Geometry: see drawing. Coordinates: mm, zero at the bounding-box minimum. Coordinates: 2 decimals unless noted, no trailing zeros. Order: outer loops, then holes, each group sorted by start corner. A loop starts at its lowest first (then second) coordinate and runs counter-clockwise, first axis right, second up. Notation, with made-up numbers: (69, 28) - (121, 28) arc R10 cw to (121, 42) - close; hole circle Ø3 at (21, 27.25). An arc over 180 degrees is marked (long way). Use a Markdown table: item, result. Add a question column.
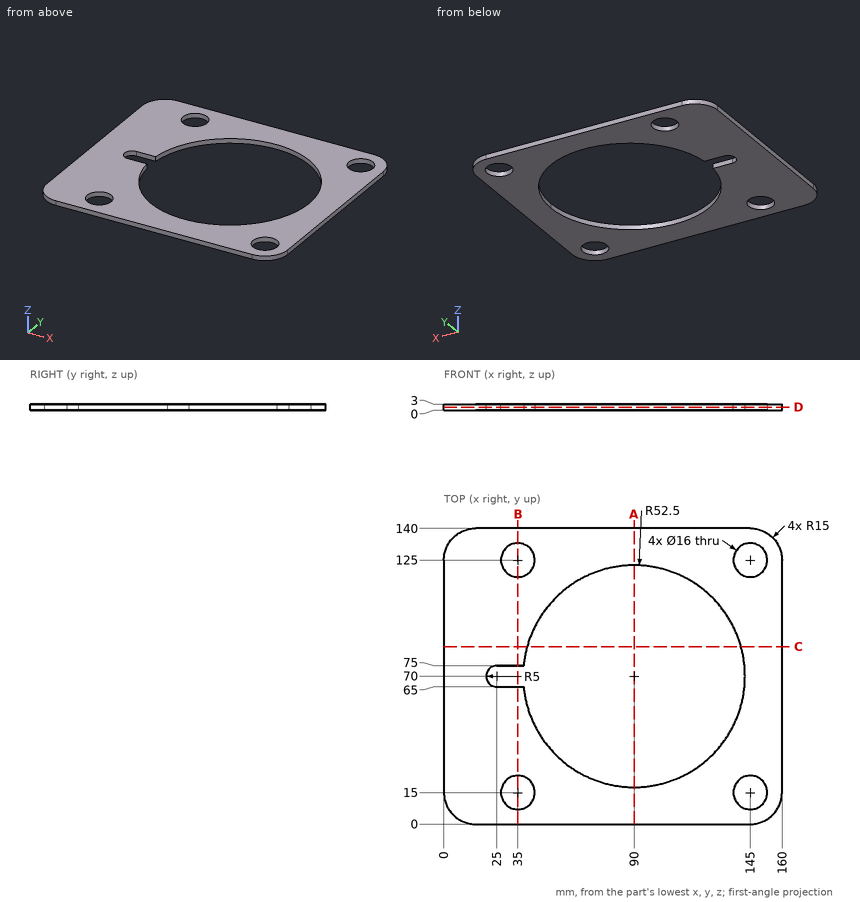
1) Line query: line 1 (Y direction, x = 145, z = 2.05); line 2 (Y direction, x = 35, z = 1.95); line 3 (X direction, y = 128, z = 1.9). Output: solid intervals per line, ascending. Write a range as from..to.
2) First-contact query: pin 1 (13 mm diameter, centred on x = 145, y = 125, fed in from +Z). Flat tip, straight axial feed; report the tip coordinate or a pass-through.
3) Section query A-A (x = 90). Return the cut outline in (y, z).
4) Section query C-C (y = 84). Return the cut outline in (x, z).
5) Section query B-B (x = 35). Return the cut outline in (y, z), and give its area (3 significant figures).
6) Section query D-D (z = 1.5). Return the cut outline in (x, y), and give its area (3 significant figures).
From the geometry:
| question | item | result |
|---|---|---|
| 1 | line 1 | y = 0..7, 23..117, 133..140 |
| 1 | line 2 | y = 0..7, 23..65, 75..117, 133..140 |
| 1 | line 3 | x = 0.3..27.58, 42.42..137.58, 152.42..159.7 |
| 2 | pin 1 | passes through |
| 3 | outline | (0, 0) - (17.5, 0) - (17.5, 3) - (0, 3) - close; (122.5, 0) - (140, 0) - (140, 3) - (122.5, 3) - close |
| 4 | outline | (0, 0) - (39.4, 0) - (39.4, 3) - (0, 3) - close; (140.6, 0) - (160, 0) - (160, 3) - (140.6, 3) - close |
| 5 | outline | (0, 0) - (7, 0) - (7, 3) - (0, 3) - close; (23, 0) - (65, 0) - (65, 3) - (23, 3) - close; (75, 0) - (117, 0) - (117, 3) - (75, 3) - close; (133, 0) - (140, 0) - (140, 3) - (133, 3) - close |
| 5 | area | 294 mm^2 |
| 6 | outline | (0, 15) arc R15 ccw to (15, 0) - (145, 0) arc R15 ccw to (160, 15) - (160, 125) arc R15 ccw to (145, 140) - (15, 140) arc R15 ccw to (0, 125) - close; hole (25, 65) - (37.74, 65) arc R52.5 ccw (long way) to (37.74, 75) - (25, 75) arc R5 ccw to start; hole circle Ø16 at (35, 15); hole circle Ø16 at (35, 125); hole circle Ø16 at (145, 15); hole circle Ø16 at (145, 125) |
| 6 | area | 12,600 mm^2 |
